Check sheet for the drawn part. Datum: minimum x, y, z corner. Units: mm. A direction names the side the tool comes from. Coordinates: 2 decimals unless noted, no trailing zeros. Order: outer loops, then holes, each group sorted by start corner. A loop starts at its lowest first (then second) coordinate and runs counter-clockwise, first axis right, second up. Notation, with made-up numbers: (11, 27) - (23, 27) arc R22 ccw to (23, 52) - close; hole circle Ø7 at (87, -19.75). An arc over 180 degrees is marked (long way). Return JSON: item names as keys, results as strings. Group by question number.
Item 1: Scan lines: probe 1 along X at (y, z) = (1.25, 285.75) (3 decimals); probe 2 along Y at (x, z) = (22, 106.5) (3 decimals). Record each from-to range of solid material in increasing order.
Item 2: Gauge pin test, flat ends, axial feed: pin 1 (1.8 mm diameter, centred on x = 15.875, z = 285.75, fed in from +Y); pin 2 (11 mm diameter, centred on y = 9.5, z = 187, fed in from +X) (3 decimals); pin 3 (3 mm diameter, centred on x = 15.5, y = 3, fed in from -Z). Record the tip position at first contact, or that the pin passes through.
Item 3: Section check A-A on y = 11. Enter the section's corners in (x, z) (3 decimals).
Item 4: Tool access check on the marked faces 1 and 2. Record the directions out of +Z, -Z, +X, -X, +Y, -Y that give a thin tool (end or side, any length) a straight path to the whole face; none if there is none.
Item 5: Section check C-C on x = 10.5. Enter the section's corners in (y, z) (3 decimals).
Item 6: Section check B-B on z = 205. Enter the section's corners in (x, y) (3 decimals), then the cut area to 3 significant figures.
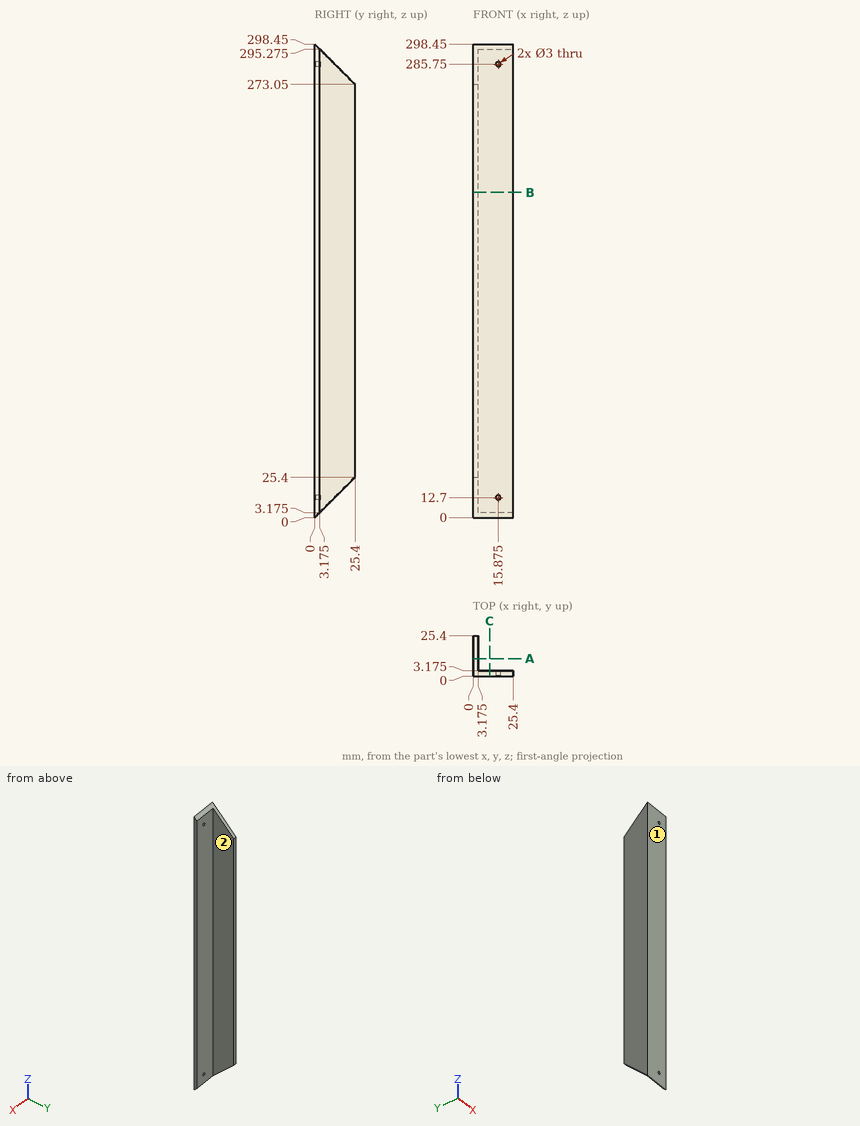
Computed:
{
 "1": {"probe 1": "x = 0 to 14.375, 17.375 to 25.4", "probe 2": "y = 0 to 3.175"},
 "2": {"pin 1": "passes through", "pin 2": "stops at x = 3.175", "pin 3": "stops at z = 1.5"},
 "3": {"outline": "(0, 11) - (3.175, 11) - (3.175, 287.45) - (0, 287.45) - close"},
 "4": {"face 1": "+Z, -Z, +X, -X, -Y", "face 2": "+Z, -Z, +X, +Y"},
 "5": {"outline": "(0, 0) - (3.175, 3.175) - (3.175, 295.275) - (0, 298.45) - close"},
 "6": {"outline": "(0, 0) - (25.4, 0) - (25.4, 3.175) - (3.175, 3.175) - (3.175, 25.4) - (0, 25.4) - close", "area": "151 mm²"}
}
